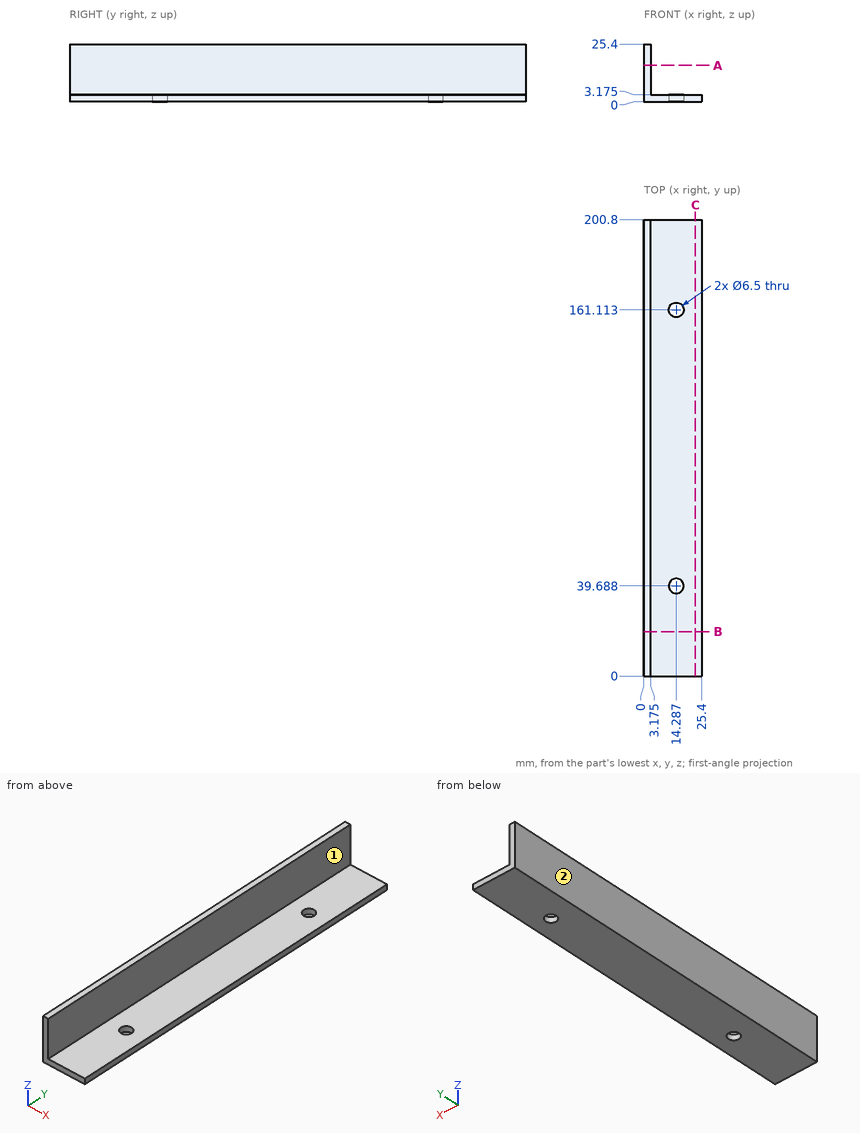
Could you check a few things on this drawing? It's one solid part, dimensions in mm from its lowest x, y, z. A direction names the side the tool comes from. Round coordinates to 2 decimals unless told otherwise and drop trailing zeros. Loops run counter-clockwise (first coordinate to the right, second up) from the corner with the lowest first, then second, coordinate; pieces in that order, holes last.
Q1. I want a section at C-C (x = 22.75). Write out the boundary of the cut face in (y, z) (1 decimal).
Q2. Please list where this line runs through material, in increasing order: L1, parallel to X at y = 148, z = 21 (1 decimal).
Q3. For P1, Ø4, axis at x = 13.5, y = 59, coming from the +Z side (1 decimal); P2, Ø6, axis at y = 97, z = 22.5, coming from the +X side (1 decimal), each with a flat end and sliding along its axis, tell me the tip position at first contact or that it passes through.
Q4. On a 3-axis mill with a long thin cutter (end or side, diameter ignored), from which of +Z, -Z, +X, -X, +Y, -Y can I reach the whole of each face in a straight line? I mean the marked faces 1 and 2. Say none if no direction works.
Q5. I want a section at B-B (y = 19.5). Write out the boundary of the cut face in (x, z) (1 decimal).
Q6. I want a section at A-A (z = 16). Write out the boundary of the cut face in (x, y) (1 decimal).
Answer below:
1. outline: (0, 0) - (200.8, 0) - (200.8, 3.2) - (0, 3.2) - close
2. L1: x = 0 to 3.2
3. P1: stops at z = 3.2
3. P2: stops at x = 3.2
4. face 1: +Z, +X, +Y, -Y
4. face 2: +Z, -Z, -X, +Y, -Y
5. outline: (0, 0) - (25.4, 0) - (25.4, 3.2) - (3.2, 3.2) - (3.2, 25.4) - (0, 25.4) - close
6. outline: (0, 0) - (3.2, 0) - (3.2, 200.8) - (0, 200.8) - close
